Check sheet for the modelled part. Datum: model origin and axes. Units: mm. Face numbers are marked on the shaded views. A direction names the side the tool comes from. Give positions to 0.01 mm unless a question says otherwise; leave off trailing zeros. Order: outer loops, then holes, each group sorted by start corner. A loop starts at its lowest first (then second) coordinate and runs counter-clockwise, first axis right, second up.
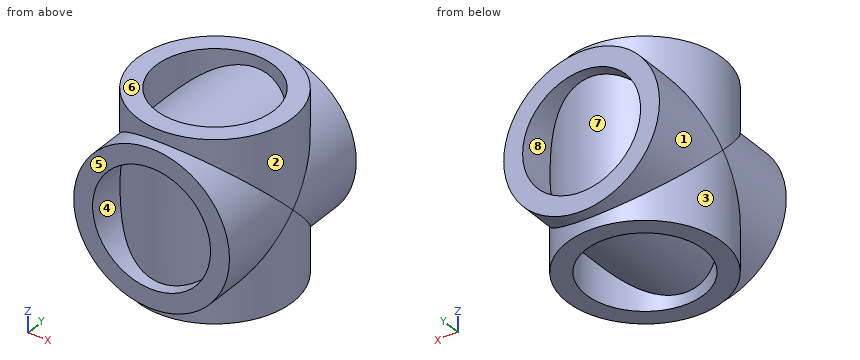
```python
from build123d import *

# Parameters (mm, degrees)
SKETCH2_R           = 8.25
SKETCH2_R_2         = 6.25
EXTRUDE_THIN1_DEPTH = 19
SKETCH4_R           = 8.25
SKETCH4_R_2         = 6.25
EXTRUDE_THIN2_DEPTH = 9.5


with BuildPart() as part:
    # Sketch2 → Extrude-Thin1 (new body)
    with BuildSketch(Plane.XY):
        Circle(SKETCH2_R)
        Circle(SKETCH2_R_2, mode=Mode.SUBTRACT)
    extrude(amount=EXTRUDE_THIN1_DEPTH)

    # Sketch4 → Extrude-Thin2 (add, symmetric)
    with BuildSketch(Plane(origin=(0, 0, 0), x_dir=(1, 0, 0), z_dir=(0, 1, 0))):
        with Locations((0, -9.5)):
            Circle(SKETCH4_R)
        with Locations((0, -9.5)):
            Circle(SKETCH4_R_2, mode=Mode.SUBTRACT)
    extrude(amount=EXTRUDE_THIN2_DEPTH, both=True)


solid = part.part
```
(1) Cross-section at B-B on z = 10.5. Enter the section's corners in (x, y), then the cut area to 3 significant figures.
Response values:
outline: (-8.19, -9.5) - (-6.17, -9.5) - (-6.17, -5.48) arc R8.25 ccw to (6.17, -5.48) - (6.17, -9.5) - (8.19, -9.5) - (8.19, -1) arc R8.25 ccw to (8.19, 1) - (8.19, 9.5) - (6.17, 9.5) - (6.17, 5.48) arc R8.25 ccw to (-6.17, 5.48) - (-6.17, 9.5) - (-8.19, 9.5) - (-8.19, 1) arc R8.25 ccw to (-8.19, -1) - close; hole (-6.17, -1) arc R6.25 ccw to (6.17, -1) - (6.17, 1) arc R6.25 ccw to (-6.17, 1) - close
area: 137 mm2
(2) Release check for a two-part mould opening along Z. For the marked faces 5, 6, 7 and 8 record: released by +Z, released by -Z, zero draft, split by the parting line, or undercut.
Response values:
face 5: zero draft
face 6: released by +Z
face 7: undercut
face 8: undercut
(3) Gauge pin test, flat ends, axial feed: pin 1 Ø2 at (x, z) = (-4.5, 11.5) entering from -Y; pin 2 Ø4 at (y, z) = (-4.5, 12) entering from -X; pin 3 Ø1 at (y, z) = (4, 16) entering from -X. Record the tip position at first contact, or that the pin passes through.
Response values:
pin 1: stops at y = -7.47
pin 2: stops at x = -8.23
pin 3: stops at x = -7.47
(4) Set-up check for the marked faces 1, 2, 3 and 4: record each of +Z, -Z, +X, -X, +Y, -Y from which the full face is reachable in a straight line by a thin tool's end or side.
Response values:
face 1: +Y
face 2: +Z
face 3: -Z
face 4: -Y
(5) Cross-section at C-C on z = 2.5. Enter the section's corners in (x, y).
Response values:
outline: (-4.37, -9.5) - (4.37, -9.5) - (4.37, -7) arc R8.25 ccw to (4.37, 7) - (4.37, 9.5) - (-4.37, 9.5) - (-4.37, 7) arc R8.25 ccw to (-4.37, -7) - close; hole (-4.37, -4.47) - (-4.37, 4.47) arc R6.25 ccw to start; hole (4.37, -4.47) arc R6.25 ccw to (4.37, 4.47) - close
(6) Material ranges on L1, parallel to Y at x = 0, z = 4.75; L2, parallel to Z at x = 0.25, y = 4.5 (3 decimals); L3, parallel to X at y = 6.95, z = 9.5, recorded low to high.
Response values:
L1: y = -8.25 to -6.25, 6.25 to 8.25
L2: z = 1.254 to 3.255, 15.745 to 17.746
L3: x = -8.25 to -6.25, -4.45 to 4.45, 6.25 to 8.25
